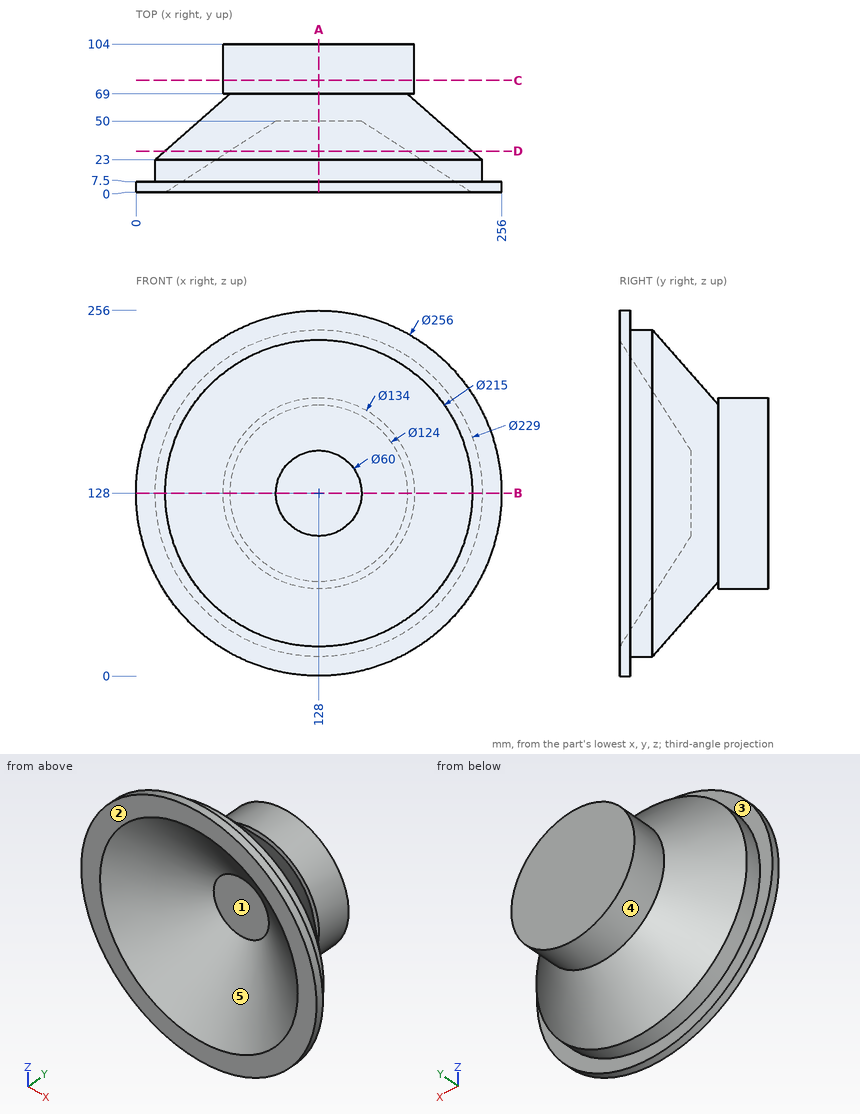
Check sheet for the drawn part. Datum: minimum x, y, z corner. Units: mm. A direction names the side the tool comes from. Round coordinates to 2 decimals unless told otherwise and drop trailing zeros. Loops run counter-clockwise (first coordinate to the right, second up) from the corner with the lowest first, then second, coordinate; pieces in that order, holes last. Notation, with made-up numbers: (-37, 83) -> (-26, 83) arc R33 ccw to (-26, 114) -> close; hole circle Ø9 at (4, 12). An arc over 180 degrees is marked (long way). Put each result on its own line as item: value. Start each with the question number.
1. Draft check along X on the marked faces 3, 4 and 5. Enter one of: +X half, -X half, draft (parallel to the pull), parting line (faces both ways), or undercut.
2. Section check C-C (y = 78.5). Enter the section's corners in (x, z), plus the area to 3 significant figures.
3. Section check D-D (y = 29). Enter the section's corners in (x, z), plus the area to 3 significant figures.
4. Section check A-A (x = 128). Enter the section's corners in (y, z).
5. Gauge pin test, flat ends, axial feed: pin 1 (4 mm diameter, centred on x = 41, z = 36, fed in from +Y); pin 2 (2 mm diameter, centred on x = 99.5, z = 168.5, fed in from -Y); pin 3 (4 mm diameter, centred on x = 51.5, z = 181.5, fed in from +Y). Record the tip position at first contact, or that the pin passes through.
6. Section check B-B (z = 128). Enter the section's corners in (x, y), plus the area to 3 significant figures.
7. Scan lines: probe 1 along X at (y, z) = (13, 139); probe 2 along X at (y, z) = (19, 174); probe 3 along Y at (x, z) = (189, 105). Record each from-to range of solid material in increasing order.
8. Access from +Z, -Z, +X, -X, +Y, -Y to the whole of each face (thin tool, end or side, straight path). Record for the marked faces 1 and 2.
Findings:
1. face 3: draft
1. face 4: parting line
1. face 5: undercut
2. outline: circle Ø134 at (128, 128)
2. area: 14,100 mm^2
3. outline: circle Ø215.3 at (128, 128); hole circle Ø125.1 at (128, 128)
3. area: 24,100 mm^2
4. outline: (0, 0) -> (7.5, 0) -> (7.5, 13.5) -> (23, 13.5) -> (69, 66) -> (69, 61) -> (104, 61) -> (104, 195) -> (69, 195) -> (69, 190) -> (23, 242.5) -> (7.5, 242.5) -> (7.5, 256) -> (0, 256) -> (0, 235.5) -> (50, 158) -> (50, 98) -> (0, 20.5) -> close
5. pin 1: stops at y = 7.5
5. pin 2: stops at y = 36.76
5. pin 3: stops at y = 43.28
6. outline: (0, 0) -> (20.5, 0) -> (98, 50) -> (158, 50) -> (235.5, 0) -> (256, 0) -> (256, 7.5) -> (242.5, 7.5) -> (242.5, 23) -> (190, 69) -> (195, 69) -> (195, 104) -> (61, 104) -> (61, 69) -> (66, 69) -> (13.5, 23) -> (13.5, 7.5) -> (0, 7.5) -> close
6. area: 11,400 mm^2
7. probe 1: x = 14.03 to 41.35, 214.65 to 241.97
7. probe 2: x = 23.15 to 64.95, 191.05 to 232.85
7. probe 3: y = 27.3 to 66.2, 69 to 104
8. face 1: -Y
8. face 2: +Z, -Z, +X, -X, -Y
